CAD build for the part. Positions are in the model's coordinates, mm. A direction names the side the tool comes from. Coordinates: 2 decimals unless noted, no trailing zeros. Order: outer loops, then holes, each group sorted by start corner. A loop starts at its lowest first (then second) coordinate and runs counter-clockwise, first axis right, second up. Notation, with made-up numbers: (-39, 18.5) - (7, 18.5) arc R17 cw to (7, 22.5) - close; hole circle Ø2 at (37.5, -17.5). An arc over 180 degrees is marked (long way). Return JSON: item names as keys, results as strings.
from build123d import *

# Parameters (mm, degrees)
CUT_EXTRUDE_1_DEPTH      = 37.701498607
PATTERN_CIRCULAR_1_COUNT = 8
SKETCH_14_R              = 6
CUT_EXTRUDE_5_DEPTH      = 28
SKETCH_15_R              = 11
CUT_EXTRUDE_6_DEPTH      = 6
CUT_EXTRUDE_7_DEPTH      = 37.701498779
CUT_EXTRUDE_7_DEPTH_BACK = 37.701498779


with BuildPart() as part:
    # 草图4 → 旋转1 (revolve)
    with BuildSketch(Plane(origin=(0, 0, 0), x_dir=(0, 0, -1), z_dir=(1, 0, 0))):
        with BuildLine():
            Line((0, 10), (-17.8, 10))
            Line((-17.8, 10), (-17.8, 13.333431373))
            ThreePointArc((-17.8, 13.333431373), (-18.129167352, 16.240319744), (-19.1, 19))
            Line((-19.1, 19), (-23.7, 19))
            ThreePointArc((-23.7, 19), (-24.670832648, 16.240319744), (-25, 13.333431373))
            Line((-25, 13.333431373), (-25, 5))
            Line((-25, 5), (0, 5))
            Line((0, 5), (0, 10))
        make_face()
    revolve(axis=Axis((0, 0, 0), (0, 0, 1)))

    # 草图5 → 切除-拉伸1 (cut, through all)
    with BuildSketch(Plane.XY):
        with BuildLine():
            Line((0.65, 18.988878324), (2.31192381, 13.985375154))
            ThreePointArc((2.31192381, 13.985375154), (4.721353225, 11.395659205), (8.256304086, 11.522549751))
            Line((8.256304086, 11.522549751), (12.969867869, 13.884614776))
            ThreePointArc((12.969867869, 13.884614776), (7.272453285, 17.553102951), (0.65, 18.988878324))
        make_face()
    cut_extrude_1 = extrude(amount=CUT_EXTRUDE_1_DEPTH, mode=Mode.SUBTRACT)

    # 阵列(圆周)1: 切除-拉伸1 ×8 about axis
    pattern_circular_1_axis = Axis((0, 0, 0), (0, 0, 1))
    for i in range(1, PATTERN_CIRCULAR_1_COUNT):
        add(cut_extrude_1.rotate(pattern_circular_1_axis, i * 360 / PATTERN_CIRCULAR_1_COUNT), mode=Mode.SUBTRACT)

    # 草图14 → 切除-拉伸5 (cut)
    with BuildSketch(Plane.XY.offset(25)):
        Circle(SKETCH_14_R)
    extrude(amount=-CUT_EXTRUDE_5_DEPTH, mode=Mode.SUBTRACT)

    # 草图15 → 切除-拉伸6 (cut)
    with BuildSketch(Plane.XY.offset(25)):
        Circle(SKETCH_15_R)
    extrude(amount=-CUT_EXTRUDE_6_DEPTH, mode=Mode.SUBTRACT)

    # 草图16 → 切除-拉伸7 (cut, two sides: drawn at the far end of the back side and taken through both)
    with BuildSketch(Plane(origin=(0, 0, 0), x_dir=(1, 0, 0), z_dir=(0, 1, 0)).offset(-CUT_EXTRUDE_7_DEPTH_BACK)):
        Polygon((-109.354391609, -14.859816975), (-15.287230377, -16.039870969), (19.672911223, -16.478439053), (113.740072455, -17.658493047), (116.100180443, 170.475829416), (-106.994283621, 173.274505489), align=None)
    extrude(amount=CUT_EXTRUDE_7_DEPTH + CUT_EXTRUDE_7_DEPTH_BACK, mode=Mode.SUBTRACT)


solid = part.part
Item 1: Which spindle directions (+Z, -Z, +X, -X, +Y, -Y) get a long thin tool onto all of the face, cutting with end or side? Do faces 1 (the cylindrical face through (13.43, -13.44, 21.43)), 2 (the flat face through (10, -5, 25)), 3 (the flat face through (-10.58, -12.687, 21.35)), 4 (the flat face through (5, -9, 17.8)), 5 (the flat face through (-12.7, -10.6, 21.3)). Say none if no direction does.
Findings below:
{"face 1": "+Z, -Z, +X, -Y", "face 2": "+Z, +X, -X, +Y, -Y", "face 3": "+Z, -Z, -Y", "face 4": "-Z", "face 5": "+Z, -Z, -X"}
Item 2: Band-saw the part on C-C, the plane z = 17. List the corners of the cut face in (x, y).
Findings below:
{"outline": "circle Ø20 at (0, 0); hole circle Ø12 at (0, 0)"}
Item 3: Band-saw the part on D-D, the plane x = 0. List the corners of the cut face in (y, z), then the cut area to 3 significant figures.
Findings below:
{"outline": "(-19, 19.1) arc R13 ccw to (-13.33, 17.8) - (-10, 17.8) - (-10, 16.23) - (-6, 16.23) - (-6, 19) - (-11, 19) - (-11, 25) - (-13.33, 25) arc R13 ccw to (-19, 23.7) - close; (6, 16.23) - (10, 16.23) - (10, 17.8) - (13.33, 17.8) arc R13 ccw to (19, 19.1) - (19, 23.7) arc R13 ccw to (13.33, 25) - (11, 25) - (11, 19) - (6, 19) - close", "area": "130 mm²"}
Item 4: Band-saw the part on A-A, the plane x = 5.5. List the corners of the cut face in (y, z), then the cut area to 3 significant figures.
Findings below:
{"outline": "(-11.16, 17.8) - (-8.35, 17.8) - (-8.35, 16.3) - (-2.4, 16.3) - (-2.4, 19) - (-9.53, 19) - (-9.53, 25) - (-11.16, 25) - close; (2.4, 16.3) - (8.35, 16.3) - (8.35, 17.8) - (11.16, 17.8) - (11.16, 25) - (9.53, 25) - (9.53, 19) - (2.4, 19) - close", "area": "58.5 mm²"}
Item 5: Wall check: L1, parallel to Y at x = 0, z = 22.4; L2, parallel to Y at x = -11.5, z = 22.25; L3, parallel to X at y = 0, z = 17.7. Give the ranges that are in metal, low to high. Write a range as [from, to].
Findings below:
{"L1": "y = [-19, -11], [11, 19]", "L2": "y = [-13.15, -8.21], [-4.49, 4.49], [8.21, 13.15]", "L3": "x = [-10, -6], [6, 10]"}
Item 6: Mould opens along X. For faces 6 (the cylindrical face through (-4.767, 11.377, 21.35)), 7 (the flat face through (16.52, -1.47, 21.35)), 8 (the cylindrical face through (-11.377, -4.767, 21.35)), 9 (the flat face through (10.6, -12.7, 21.3)) say: released by +X, released by -X, zero draft, split by the parting line, or undercut.
Findings below:
{"face 6": "undercut", "face 7": "released by +X", "face 8": "released by -X", "face 9": "undercut"}
Item 7: Band-saw the part on B-B, the plane y = 0. List the corners of the cut face in (x, z), then the cut area to 3 significant figures.
Findings below:
{"outline": "(-19, 19.1) arc R13 ccw to (-13.33, 17.8) - (-10, 17.8) - (-10, 16.11) - (-6, 16.16) - (-6, 19) - (-11, 19) - (-11, 25) - (-13.33, 25) arc R13 ccw to (-19, 23.7) - close; (6, 16.31) - (10, 16.36) - (10, 17.8) - (13.33, 17.8) arc R13 ccw to (19, 19.1) - (19, 23.7) arc R13 ccw to (13.33, 25) - (11, 25) - (11, 19) - (6, 19) - close", "area": "130 mm²"}
Item 8: Drop flat-ended pins along their axis: P1, Ø5, axis at x = -4.5, y = 7, coming from the -Z side; P2, Ø1, axis at y = 13.5, z = 24, coming from the +X side; P3, Ø17.5, axis at x = 0, y = 0, coming from the +Z side. Give the stop position or say it passes through.
Findings below:
{"P1": "stops at z = 16.14", "P2": "stops at x = 13.76", "P3": "stops at z = 19"}
